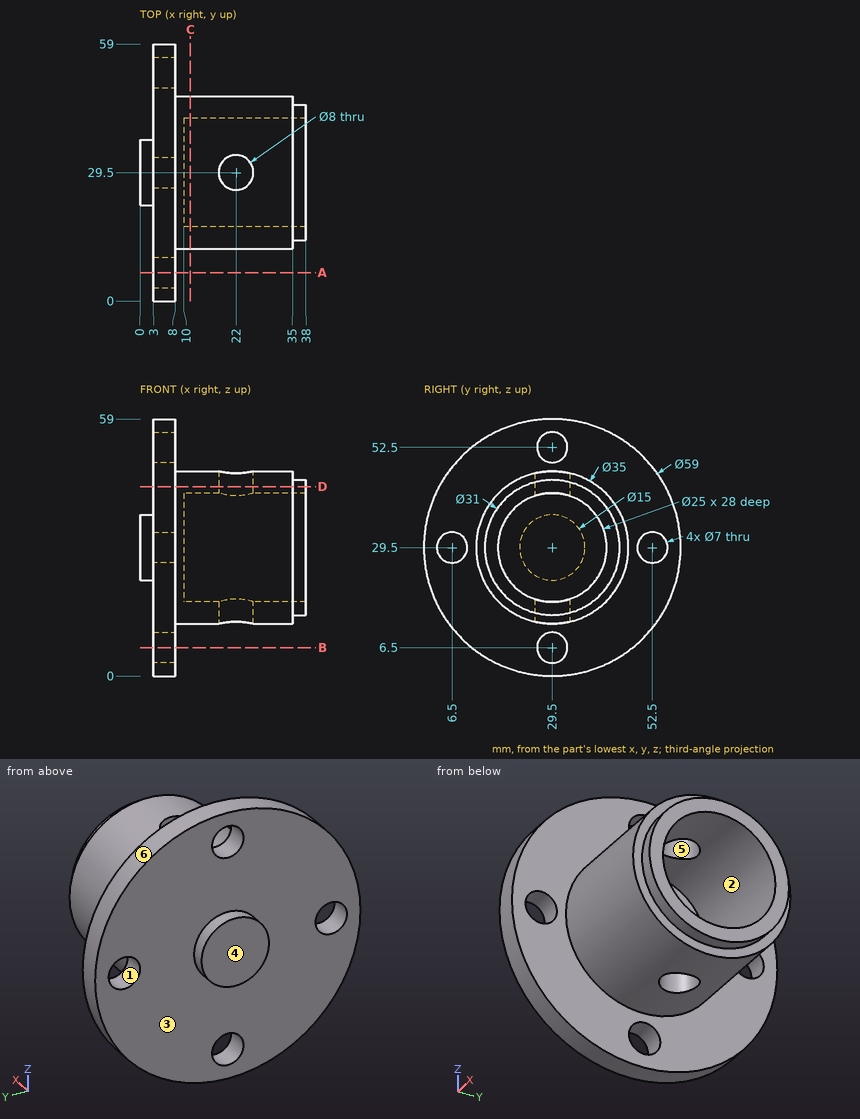
Study the drawing (mm; zero at the part's minimum x, y, z) and answer. A direction names the side the tool comes from. Give positions to 0.01 mm unless a question says otherwise; leave off trailing zeros. Loops run counter-clockwise (first coordinate to the right, second up) from the corner with the lowest first, then second, coordinate; pieces in that order, holes last. Notation, with made-up numbers: (-32.75, 58) - (-4.75, 58) arc R23 cw to (-4.75, 83) - close; hole circle Ø8 at (7.25, 47.5). An arc over 180 degrees is marked (long way). Answer in a Markdown table with one row per item. Add a question column.
Q1. The part is cut by section A-A (y = 6.5). Determine the outline of the cut face in (x, z), and give its area (3 significant figures).
Q2. The part is cut by section C-C (x = 11.5). Determine the outline of the cut face in (y, z), and give its area (3 significant figures).
Q3. Consider line 1 along Z through (x, y) = (4, 29); line 2 along X through (y, z) = (39, 27); line 3 along Z through (x, y) = (32.5, 41). Determine where each line is inside the solid, lowest interval first.
Q4. A tool of negligible diameter and unlimited length cuts with its end or side. For the marked faces 1, 2 and 3, from which of +Z, -Z, +X, -X, +Y, -Y can it reach the whole face along a straight path? Write none if from no direction.
Q5. Determine the mould class of the marked faces 4, 5 and 6 for opening direction Y: released by +Y, released by -Y, zero draft, split by the parting line, or undercut.
Q6. Each of these flat-tipped pins is pushed along its axis until it touches: P1, Ø2, axis at y = 10, z = 22.5, coming from the +X side; P2, Ø10, axis at x = 7, y = 43, coming from the -Z side; P3, Ø5, axis at x = 25.5, z = 24, coming from the -Y side. Where does it stop, or does it pass through?
Q7. The part is cut by section D-D (z = 43.5). Determine the outline of the cut face in (x, y).
Solution:
| question | item | result |
|---|---|---|
| 1 | outline | (3, 11.03) - (8, 11.03) - (8, 26) - (3, 26) - close; (3, 33) - (8, 33) - (8, 47.97) - (3, 47.97) - close |
| 1 | area | 150 mm² |
| 2 | outline | circle Ø35 at (29.5, 29.5); hole circle Ø25 at (29.5, 29.5) |
| 2 | area | 471 mm² |
| 3 | line 1 | z = 0 to 3.04, 9.96 to 49.04, 55.96 to 59 |
| 3 | line 2 | x = 3 to 10 |
| 3 | line 3 | z = 16.31 to 24.6, 34.4 to 42.69 |
| 4 | face 1 | +X, -X |
| 4 | face 2 | +X |
| 4 | face 3 | -X |
| 5 | face 4 | zero draft |
| 5 | face 5 | undercut |
| 5 | face 6 | split by the parting line |
| 6 | P1 | stops at x = 8 |
| 6 | P2 | stops at z = 1.25 |
| 6 | P3 | stops at y = 12.26 |
| 7 | outline | (3, 3.53) - (8, 3.53) - (8, 19) - (35, 19) - (35, 22.85) - (38, 22.85) - (38, 36.15) - (35, 36.15) - (35, 40) - (8, 40) - (8, 55.47) - (3, 55.47) - close; hole circle Ø8 at (22, 29.5) |
